from build123d import *

# Parameters (mm, degrees)
EXTRUDE_1_DEPTH = 1
EXTRUDE_2_DEPTH = 7
SKETCH_5_W      = 1
SKETCH_5_H      = 27
EXTRUDE_3_DEPTH = 1.5
SKETCH_7_W      = 1
SKETCH_7_H      = 27
EXTRUDE_4_DEPTH = 1.5
SKETCH_8_W      = 28
SKETCH_8_H      = 28
EXTRUDE_5_DEPTH = 1


with BuildPart() as part:
    # 스케치1 → 보스-돌출1 (new body)
    with BuildSketch(Plane.XY):
        Polygon((20, 0), (28, 0), (28, -28), (0, -28), (0, 0), (8, 0), (8, -23), (20, -23), align=None)
    extrude(amount=EXTRUDE_1_DEPTH)

    # 스케치3 → 보스-돌출2 (add)
    with BuildSketch(Plane.XY.offset(1)):
        Polygon((1, 0), (0, 0), (0, -28), (28, -28), (28, 0), (27, 0), (27, -27), (1, -27), align=None)
    extrude(amount=EXTRUDE_2_DEPTH)

    # 스케치5 → 보스-돌출3 (add)
    with BuildSketch(Plane(origin=(1, 0, 0), x_dir=(0, 0, -1), z_dir=(1, 0, 0))):
        with Locations((-2.5, -13.5)):
            Rectangle(SKETCH_5_W, SKETCH_5_H)
    extrude(amount=EXTRUDE_3_DEPTH)

    # 스케치7 → 보스-돌출4 (add)
    with BuildSketch(Plane.ZY.offset(-27)):
        with Locations((2.5, -13.5)):
            Rectangle(SKETCH_7_W, SKETCH_7_H)
    extrude(amount=EXTRUDE_4_DEPTH)

    # 스케치8 → 보스-돌출5 (add)
    with BuildSketch(Plane.XY.offset(8)):
        with Locations((14, -14)):
            Rectangle(SKETCH_8_W, SKETCH_8_H)
    extrude(amount=EXTRUDE_5_DEPTH)


solid = part.part
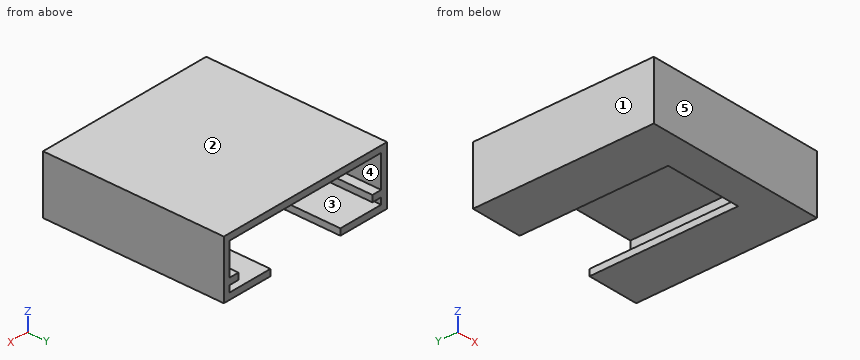
The model under review builds one solid part; all positions refer to its coordinate system, in mm. Face numbers are marked on the shaded views. A direction names the side the tool comes from. Round coordinates to 2 decimals unless told otherwise and drop trailing zeros. Order: outer loops, then holes, each group sorted by start corner. A loop starts at its lowest first (then second) coordinate and runs counter-clockwise, first axis right, second up. Notation, with made-up numbers: (-31.75, -34) - (17.25, -34) arc R21 cw to (17.25, 4) - close; hole circle Ø6 at (-36.5, -14). An arc over 180 degrees is marked (long way). Use one line per item in the form item = value.
Q1. Mouldability with a two-part tool opening along X and no side actions: class the marked faces 1, 2 and 3 as pulls with the +X half, pulls with the -X half, needs draft (parallel to the pull), parting line crosses it, or undercut.
Response values:
face_1 = pulls with the -X half
face_2 = needs draft
face_3 = undercut
Q2. To check wall thickness, follow line 1 (Z direction, x = 4.75, y = -16); line 2 (X direction, y = -24.5, z = 6); line 3 (Z direction, x = 18.75, y = -13.25). State the ranges of each line that lie inside material, in increasing order.
Response values:
line_1 = 0 to 1, 8 to 9
line_2 = 0 to 1, 27 to 28
line_3 = 8 to 9
Q3. Add section A-A on y = -2.75. Give the boundary of the cut face in (x, z), then the cut area to 3 significant figures.
Response values:
outline = (0, 0) - (8, 0) - (8, 1) - (1, 1) - (1, 2) - (2.5, 2) - (2.5, 3) - (1, 3) - (1, 8) - (27, 8) - (27, 3) - (25.5, 3) - (25.5, 2) - (27, 2) - (27, 1) - (20, 1) - (20, 0) - (28, 0) - (28, 9) - (0, 9) - close
area = 61.0 mm^2
Q4. Tool access review of the marked faces 4 and 5: name each direction out of +Z, -Z, +X, -X, +Y, -Y from which nothing blocks a thin tool from reaching the whole face with its end or side.
Response values:
face_4 = +Y
face_5 = +Z, -Z, +X, -X, -Y
Q5. Clearance check with flat-ended pins moving along their axes: P1, Ø3.5, axis at x = 8, z = 3.5, coming from the +Y side; P2, Ø4, axis at x = 10.5, y = -13.5, coming from the -Z side. State where each tip first meets the part, or that it passes through.
Response values:
P1 = -27
P2 = 8
Q6. Add section B-B on x = 6.25. Give the boundary of the cut face in (y, z), then the cut area to 3 significant figures.
Response values:
outline = (-28, 0) - (0, 0) - (0, 1) - (-27, 1) - (-27, 8) - (0, 8) - (0, 9) - (-28, 9) - close
area = 63.0 mm^2
Q7. Add section C-C on z = 5.5. Give the boundary of the cut face in (x, y), then the cut area to 3 significant figures.
Response values:
outline = (0, -28) - (28, -28) - (28, 0) - (27, 0) - (27, -27) - (1, -27) - (1, 0) - (0, 0) - close
area = 82.0 mm^2
